Could you check a few things on this model? Use its own coordinates, in mm. Coordinates: 2 decimals unless noted, no trailing zeros. Put each result on its own line as item: value. Start each with the question number.
```python
from build123d import *

# Parameters (mm, degrees)
SKETCH_1_R      = 1.6
SKETCH_1_R_2    = 3.5
EXTRUDE_1_DEPTH = 3


with BuildPart() as part:
    # 草图1 → 凸台-拉伸1 (new body)
    with BuildSketch(Plane(origin=(0, 0, 0), x_dir=(1, 0, 0), z_dir=(0, 1, 0))):
        with BuildLine():
            Line((46.95, -4), (83.804594146, -4))
            Line((83.804594146, -4), (93.814764296, -4))
            ThreePointArc((93.814764296, -4), (0, 93.9), (-93.814764296, -4))
            Line((-93.814764296, -4), (-83.804594146, -4))
            Line((-83.804594146, -4), (-46.95, -4))
            Line((-46.95, -4), (-15.491933385, -4))
            ThreePointArc((-15.491933385, -4), (0, -16), (15.491933385, -4))
            Line((15.491933385, -4), (46.95, -4))
        make_face()
        with Locations(Location((88.9, 0, 0), (0, 0, 270))):
            Circle(SKETCH_1_R, mode=Mode.SUBTRACT)
        with Locations(Location((-88.9, 0, 0), (0, 0, 270))):
            Circle(SKETCH_1_R, mode=Mode.SUBTRACT)
        with Locations(Location((-62.861792847, 62.861792847, 0), (0, 0, 270))):
            Circle(SKETCH_1_R, mode=Mode.SUBTRACT)
        with Locations(Location((0, 88.9, 0), (0, 0, 270))):
            Circle(SKETCH_1_R, mode=Mode.SUBTRACT)
        with Locations(Location((62.861792847, 62.861792847, 0), (0, 0, 270))):
            Circle(SKETCH_1_R, mode=Mode.SUBTRACT)
        with Locations(Location((0, 0, 0), (0, 0, 270))):
            Circle(SKETCH_1_R_2, mode=Mode.SUBTRACT)
        with BuildLine():
            Line((46.95, 4), (47.760369555, 4))
            ThreePointArc((47.760369555, 4), (55.764412134, 8.005393892), (57.356586062, 16.812939522))
            ThreePointArc((57.356586062, 16.812939522), (42.263772312, 42.263772312), (16.812939522, 57.356586062))
            ThreePointArc((16.812939522, 57.356586062), (8.005393892, 55.764412134), (4, 47.760369555))
            Line((4, 47.760369555), (4, 46.95))
            Line((4, 46.95), (4, 43.500766957))
            ThreePointArc((4, 43.500766957), (5.154045583, 37.698988024), (8.440489352, 32.780477341))
            Line((8.440489352, 32.780477341), (32.780477341, 8.440489352))
            ThreePointArc((32.780477341, 8.440489352), (37.698988024, 5.154045583), (43.500766957, 4))
            Line((43.500766957, 4), (46.95, 4))
        make_face(mode=Mode.SUBTRACT)
        with BuildLine():
            Line((-46.95, 4), (-43.500766957, 4))
            ThreePointArc((-43.500766957, 4), (-37.698988024, 5.154045583), (-32.780477341, 8.440489352))
            Line((-32.780477341, 8.440489352), (-8.440489352, 32.780477341))
            ThreePointArc((-8.440489352, 32.780477341), (-5.154045583, 37.698988024), (-4, 43.500766957))
            Line((-4, 43.500766957), (-4, 46.95))
            Line((-4, 46.95), (-4, 47.760369555))
            ThreePointArc((-4, 47.760369555), (-8.005393892, 55.764412134), (-16.812939522, 57.356586062))
            ThreePointArc((-16.812939522, 57.356586062), (-42.263772312, 42.263772312), (-57.356586062, 16.812939522))
            ThreePointArc((-57.356586062, 16.812939522), (-55.764412134, 8.005393892), (-47.760369555, 4))
            Line((-47.760369555, 4), (-46.95, 4))
        make_face(mode=Mode.SUBTRACT)
        with BuildLine():
            Line((-78.53185914, 4), (-81.679924094, 4))
            ThreePointArc((-81.679924094, 4), (-83.145024823, 4.638574331), (-83.674549835, 6.146520147))
            ThreePointArc((-83.674549835, 6.146520147), (-59.326258942, 59.326258942), (-6.146520147, 83.674549835))
            ThreePointArc((-6.146520147, 83.674549835), (-4.638574331, 83.145024823), (-4, 81.679924094))
            Line((-4, 81.679924094), (-4, 78.53185914))
            ThreePointArc((-4, 78.53185914), (-6.333499574, 72.111207209), (-12.244954243, 68.687072987))
            ThreePointArc((-12.244954243, 68.687072987), (-49.334840123, 49.334840123), (-68.687072987, 12.244954243))
            ThreePointArc((-68.687072987, 12.244954243), (-72.111207209, 6.333499574), (-78.53185914, 4))
        make_face(mode=Mode.SUBTRACT)
        with BuildLine():
            Line((4, 78.53185914), (4, 81.679924094))
            ThreePointArc((4, 81.679924094), (4.638574331, 83.145024823), (6.146520147, 83.674549835))
            ThreePointArc((6.146520147, 83.674549835), (59.326258942, 59.326258942), (83.674549835, 6.146520147))
            ThreePointArc((83.674549835, 6.146520147), (83.145024823, 4.638574331), (81.679924094, 4))
            Line((81.679924094, 4), (78.53185914, 4))
            ThreePointArc((78.53185914, 4), (72.111207209, 6.333499574), (68.687072987, 12.244954243))
            ThreePointArc((68.687072987, 12.244954243), (49.334840123, 49.334840123), (12.244954243, 68.687072987))
            ThreePointArc((12.244954243, 68.687072987), (6.333499574, 72.111207209), (4, 78.53185914))
        make_face(mode=Mode.SUBTRACT)
        with BuildLine():
            Line((-27.80675313, 7.414213562), (-7.414213562, 27.80675313))
            ThreePointArc((-7.414213562, 27.80675313), (-5.234633135, 28.240298633), (-4, 26.392539568))
            Line((-4, 26.392539568), (-4, 18.973665961))
            ThreePointArc((-4, 18.973665961), (-4.774228726, 16.301053542), (-6.857142857, 14.456126446))
            ThreePointArc((-6.857142857, 14.456126446), (-11.313708499, 11.313708499), (-14.456126446, 6.857142857))
            ThreePointArc((-14.456126446, 6.857142857), (-16.301053542, 4.774228726), (-18.973665961, 4))
            Line((-18.973665961, 4), (-26.392539568, 4))
            ThreePointArc((-26.392539568, 4), (-28.240298633, 5.234633135), (-27.80675313, 7.414213562))
        make_face(mode=Mode.SUBTRACT)
        with BuildLine():
            Line((27.80675313, 7.414213562), (7.414213562, 27.80675313))
            ThreePointArc((7.414213562, 27.80675313), (5.234633135, 28.240298633), (4, 26.392539568))
            Line((4, 26.392539568), (4, 18.973665961))
            ThreePointArc((4, 18.973665961), (4.774228726, 16.301053542), (6.857142857, 14.456126446))
            ThreePointArc((6.857142857, 14.456126446), (11.313708499, 11.313708499), (14.456126446, 6.857142857))
            ThreePointArc((14.456126446, 6.857142857), (16.301053542, 4.774228726), (18.973665961, 4))
            Line((18.973665961, 4), (26.392539568, 4))
            ThreePointArc((26.392539568, 4), (28.240298633, 5.234633135), (27.80675313, 7.414213562))
        make_face(mode=Mode.SUBTRACT)
        with BuildLine():
            Line((5.939696962, -8.202438662), (3.111269837, -5.374011537))
            ThreePointArc((3.111269837, -5.374011537), (3.111269837, -3.111269837), (5.374011537, -3.111269837))
            Line((5.374011537, -3.111269837), (8.202438662, -5.939696962))
            ThreePointArc((8.202438662, -5.939696962), (8.202438662, -8.202438662), (5.939696962, -8.202438662))
        make_face(mode=Mode.SUBTRACT)
        with BuildLine():
            Line((-8.202438662, -5.939696962), (-5.374011537, -3.111269837))
            ThreePointArc((-5.374011537, -3.111269837), (-3.111269837, -3.111269837), (-3.111269837, -5.374011537))
            Line((-3.111269837, -5.374011537), (-5.939696962, -8.202438662))
            ThreePointArc((-5.939696962, -8.202438662), (-8.202438662, -8.202438662), (-8.202438662, -5.939696962))
        make_face(mode=Mode.SUBTRACT)
        with BuildLine():
            Line((-5.939696962, 8.202438662), (-3.111269837, 5.374011537))
            ThreePointArc((-3.111269837, 5.374011537), (-3.111269837, 3.111269837), (-5.374011537, 3.111269837))
            Line((-5.374011537, 3.111269837), (-8.202438662, 5.939696962))
            ThreePointArc((-8.202438662, 5.939696962), (-8.202438662, 8.202438662), (-5.939696962, 8.202438662))
        make_face(mode=Mode.SUBTRACT)
        with BuildLine():
            Line((8.202438662, 5.939696962), (5.374011537, 3.111269837))
            ThreePointArc((5.374011537, 3.111269837), (3.111269837, 3.111269837), (3.111269837, 5.374011537))
            Line((3.111269837, 5.374011537), (5.939696962, 8.202438662))
            ThreePointArc((5.939696962, 8.202438662), (8.202438662, 8.202438662), (8.202438662, 5.939696962))
        make_face(mode=Mode.SUBTRACT)
    extrude(amount=EXTRUDE_1_DEPTH)


solid = part.part
```
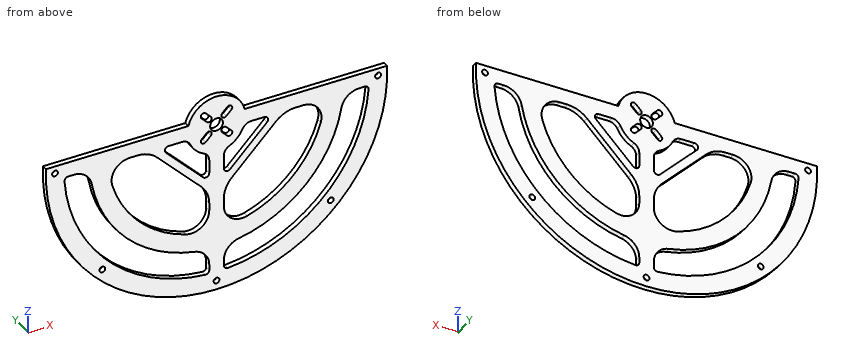
(1) I want a section at A-A on y = 2.45. Count the separate pieces of the cut face and the enclosed holes in it, and give its area (3 significant figures).
(2) I need wall thicknesses on L1, parallel to X at y = 1.85, z = 0; L2, parallel to X at y = 0.45, z = -45; L3, parallel to Z at x = 40, y = 1.8. Which ranges of each line are inside material? Lowest first, please. Write a range as [from, to].
(3) For pin 1 Ø4 at (x, z) = (0, 0) entering from +Y; pin 2 Ø1.5 at (x, y) = (-24.5, 1.5) entering from -Z; pin 3 Ø0.9 at (y, z) = (1, -45.5) entering from -X; pin 4 Ø0.9 at (x, y) = (44.5, 1.5) entering from +Z, each with a flat end and sliding along its axis, tell me the tip position at first contact or that it passes through.
Answer sheet:
1. separate pieces: 1
1. enclosed holes: 16
1. area: 7,640 mm^2
2. L1: x = [-93.9, -90.5], [-87.3, -3.5], [3.5, 87.3], [90.5, 93.9]
2. L2: x = [-82.41, -70.81], [-53.32, -39.34], [-4, 4], [39.34, 53.32], [70.81, 82.41]
2. L3: z = [-84.95, -73.75], [-57.17, -44.41], [-4.41, 4]
3. pin 1: passes through
3. pin 2: stops at z = -90.85
3. pin 3: stops at x = -82.39
3. pin 4: stops at z = 4
